```python
from build123d import *

# Parameters (mm, degrees)
BOSS_EXTRUDE1_DEPTH = 80


with BuildPart() as part:
    # Sketch1 → Boss-Extrude1 (new body)
    with BuildSketch(Plane(origin=(0, 0, 0), x_dir=(1, 0, 0), z_dir=(0, 1, 0))):
        Polygon((0, 33.721419827), (0, 62.5), (-26.364467654, 21.024961366), (-48.864467654, 38.968112616), (-32.875953428, -7.503721834), (-60.932994511, -13.907558372), (-14.631175723, -30.381949446), (-27.117733695, -56.310554244), (14.631175723, -30.381949446), (27.117733695, -56.310554244), (32.875953428, -7.503721834), (60.932994511, -13.907558372), (26.364467654, 21.024961366), (48.864467654, 38.968112616), align=None)
        with BuildLine():
            Line((-4, 17.036725037), (-4, 21.036725037))
            Line((-4, 21.036725037), (4, 21.036725037))
            Line((4, 21.036725037), (4, 17.036725037))
            ThreePointArc((4, 17.036725037), (0, -17.5), (-4, 17.036725037))
        make_face(mode=Mode.SUBTRACT)
    extrude(amount=BOSS_EXTRUDE1_DEPTH)


solid = part.part
```
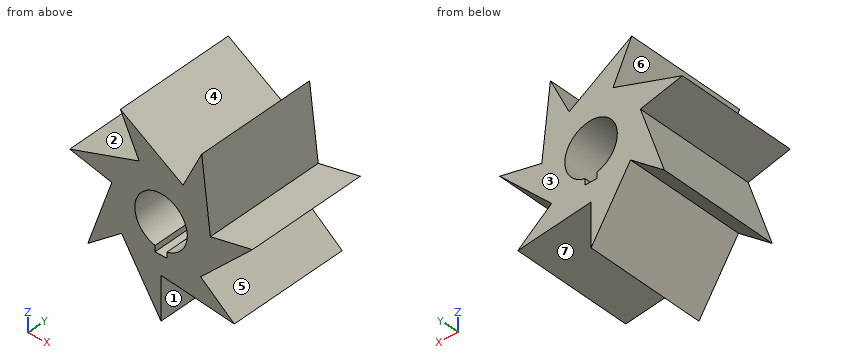
Part model, mm, in its own coordinate system. Face numbers are marked on the shaded views. A direction names the side the tool comes from. Round coordinates to 2 decimals unless told otherwise and drop trailing zeros. Write each loop counter-clockwise with the first axis right and the second up, starting at its lowest first coordinate (ties: lowest second). Pieces come first, ordered by that corner, then holes. Notation, with made-up numbers: M 59,-9.5 L 90,-9.5 A22 ccw 90,10.5 Z; hole C -2,-28.5 d2. An arc over 180 degrees is marked long. Answer as CSV lines item,"result". Start each with the question number.
1) Drop flat-ended pins along their axis: pin 1 (12 mm diameter, centred on x = 13.5, y = 18.5, fed in from +Z); pin 2 (12 mm diameter, centred on x = -31, y = 60, fed in from -Z); pin 3 (8 mm diameter, centred on y = 50.5, z = 8, fed in from +X); pin 4 (1.5 mm diameter, centred on x = 9.5, z = 11.5, fed in from -Y). Give the stop position or say it passes through.
2) Band-saw the part on C-C (x = 36.5). List the corners of the cut face in (y, z).
3) Band-saw the part on D-D (z = 27.5). List the corners of the cut face in (x, y), then the cut area to 3 significant figures.
4) Which spindle directions (+Z, -Z, +X, -X, +Y, -Y) get a long thin tool onto all of the face, cutting with end or side? Do the marked faces 4, 5, 6 and 7. Say none if no direction does.
5) Mould opens along X. For the marked faces 1, 2 and 3 say: +X half, -X half, draft (parallel to the pull), parting line (faces both ways), or undercut.
6) Band-saw the part on B-B (z = 0). List the corners of the cut face in (x, y), then the cut area to 3 significant figures.
7) Drill centre lines: L1, parallel to Z at x = -19.5, y = 35; L2, parallel to X at y = 71, z = 45; L3, parallel to X at y = 8, z = -39.5. Where is each one in solid material? Low to high.
8) Band-saw the part on A-A (y = 14). List the corners of the cut face in (x, z).
Worked out:
1,pin 1,"z = 40.49"
1,pin 2,"z = -29.51"
1,pin 3,"x = 59.05"
1,pin 4,"through"
2,outline,"M 0,-37.64 L 80,-37.64 L 80,-29.11 L 0,-29.11 Z; M 0,-10.78 L 80,-10.78 L 80,8.33 L 0,8.33 Z"
3,outline,"M -22.73,0 L 30.52,0 L 30.52,80 L -22.73,80 Z"
3,area,"4,260 mm²"
4,face 4,"+Z, +Y, -Y"
4,face 5,"+X, +Y, -Y"
4,face 6,"-X, +Y, -Y"
4,face 7,"-Z, +Y, -Y"
5,face 1,"undercut"
5,face 2,"-X half"
5,face 3,"draft"
6,outline,"M -35.46,0 L -17.5,0 L -17.5,80 L -35.46,80 Z; M 17.5,0 L 47.17,0 L 47.17,80 L 17.5,80 Z"
6,area,"3,810 mm²"
7,L1,"-31.82 to 28.65, 40.49 to 51.58"
7,L2,"-21.67 to -8.91, 21.67 to 28.45"
7,L3,"-14.62 to 0"
8,outline,"M -60.93,13.91 L -32.88,7.5 L -48.86,-38.97 L -26.36,-21.02 L 0,-62.5 L 0,-33.72 L 48.86,-38.97 L 26.36,-21.02 L 60.93,13.91 L 32.88,7.5 L 27.12,56.31 L 14.63,30.38 L -27.12,56.31 L -14.63,30.38 Z; hole M -4,-21.04 L 4,-21.04 L 4,-17.04 A17.5 ccw long -4,-17.04 Z"
